Geometry: see drawing. Coordinates: mm, zero at the bounding-box minimum. A direction names the side the tool comes from. Give positions to 0.01 mm unless a question says otherwise; leave off trailing zeros. Write each loop counter-clockwise with the first axis right and the second up, starting at its lowest first coordinate (ties: lowest second). Pieces come first, ordered by that corner, then holes. Notation, with made-up numbers: (65, 60.25) -> (113, 60.25) arc R23 ccw to (113, 98.25) -> close; hole circle Ø5 at (-10, 70.5). An arc over 180 degrees is marked (long way). Use one line per item in the form item = value. Start each with the question number.
(1) First-contact query: P1, Ø2.5, axis at x = 3, z = 3, coming from the +Y side; P2, Ø3.5, axis at x = 3, z = 3, coming from the +Y side. Flat tips, straight axial feed; report the tip coordinate or a pass-through.
(2) Cut plane D-D, the plane y = 5.5. Output: boundary loops of the cut face in (x, z), and give its area (3 significant figures).
(3) Cut plane A-A, the plane x = 12. Output: boundary loops of the cut face in (y, z), and give its area (3 significant figures).
(4) Cut plane C-C, the plane z = 3.5. Output: boundary loops of the cut face in (x, y).
(5) Set-up query: the marked faces 1, 2, 3 and 4. Return all of +Z, -Z, +X, -X, +Y, -Y with unobstructed straight access to the full face (end or side cutting, diameter ignored); none if empty.
(6) Draft query along X for the marked faces 5, 6 and 7. Return one class per face: pulls with the +X half, pulls with the -X half, needs draft (parallel to the pull), parting line crosses it, or undercut.
(7) Cut plane B-B, the plane y = 3. Output: boundary loops of the cut face in (x, z), and give its area (3 significant figures).
(8) Material intervals for line 1 along Y through (x, z) = (12, 2.6); line 2 along Z through (x, y) = (3, 7.85); line 3 along X through (y, z) = (7, 2.25), sorted ascending. Write a range as from..to.
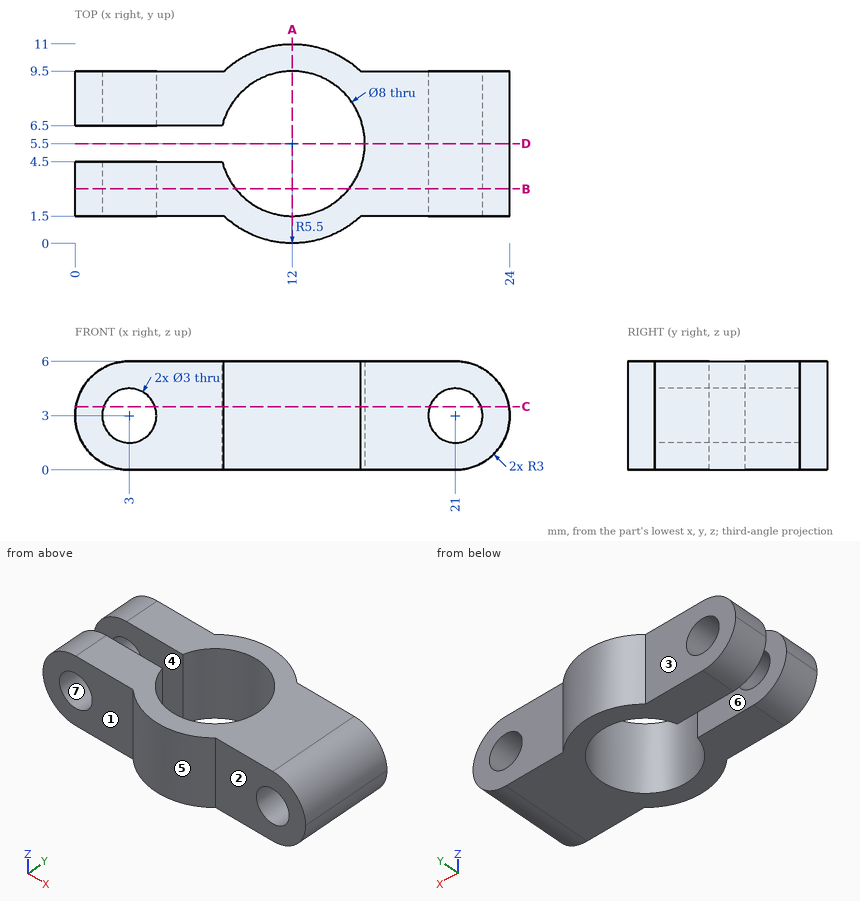
Geometry says:
q1.P1 = through
q1.P2 = 9.5
q2.outline = (16, 0) -> (21, 0) arc R3 ccw to (21, 6) -> (16, 6) -> close; hole circle Ø3 at (21, 3)
q2.area = 37.1 mm^2
q3.outline = (0, 0) -> (1.5, 0) -> (1.5, 6) -> (0, 6) -> close; (9.5, 0) -> (11, 0) -> (11, 6) -> (9.5, 6) -> close
q3.area = 18.0 mm^2
q4.outline = (0.04, 1.5) -> (1.59, 1.5) -> (1.59, 4.5) -> (0.04, 4.5) -> close; (0.04, 6.5) -> (1.59, 6.5) -> (1.59, 9.5) -> (0.04, 9.5) -> close; (4.41, 1.5) -> (8.23, 1.5) arc R5.5 ccw to (15.77, 1.5) -> (19.59, 1.5) -> (19.59, 9.5) -> (15.77, 9.5) arc R5.5 ccw to (8.23, 9.5) -> (4.41, 9.5) -> (4.41, 6.5) -> (8.13, 6.5) arc R4 cw (long way) to (8.13, 4.5) -> (4.41, 4.5) -> close; (22.41, 1.5) -> (23.96, 1.5) -> (23.96, 9.5) -> (22.41, 9.5) -> close
q5.face_1 = +Z, -Z, -X, -Y
q5.face_2 = +Z, -Z, +X, -Y
q5.face_3 = +Z, -Z, -X, +Y
q5.face_4 = +Z, -Z, -X
q6.face_5 = parting line crosses it
q6.face_6 = needs draft
q6.face_7 = undercut
q7.outline = (3, 0) -> (8.88, 0) -> (8.88, 6) -> (3, 6) arc R3 ccw to start; (15.12, 0) -> (21, 0) arc R3 ccw to (21, 6) -> (15.12, 6) -> close; hole circle Ø3 at (3, 3); hole circle Ø3 at (21, 3)
q7.area = 84.7 mm^2
q8.line_1 = 0..1.5, 9.5..11
q8.line_2 = 0..1.5, 4.5..6
q8.line_3 = 0.1..1.7, 4.3..8.29, 15.71..19.7, 22.3..23.9
